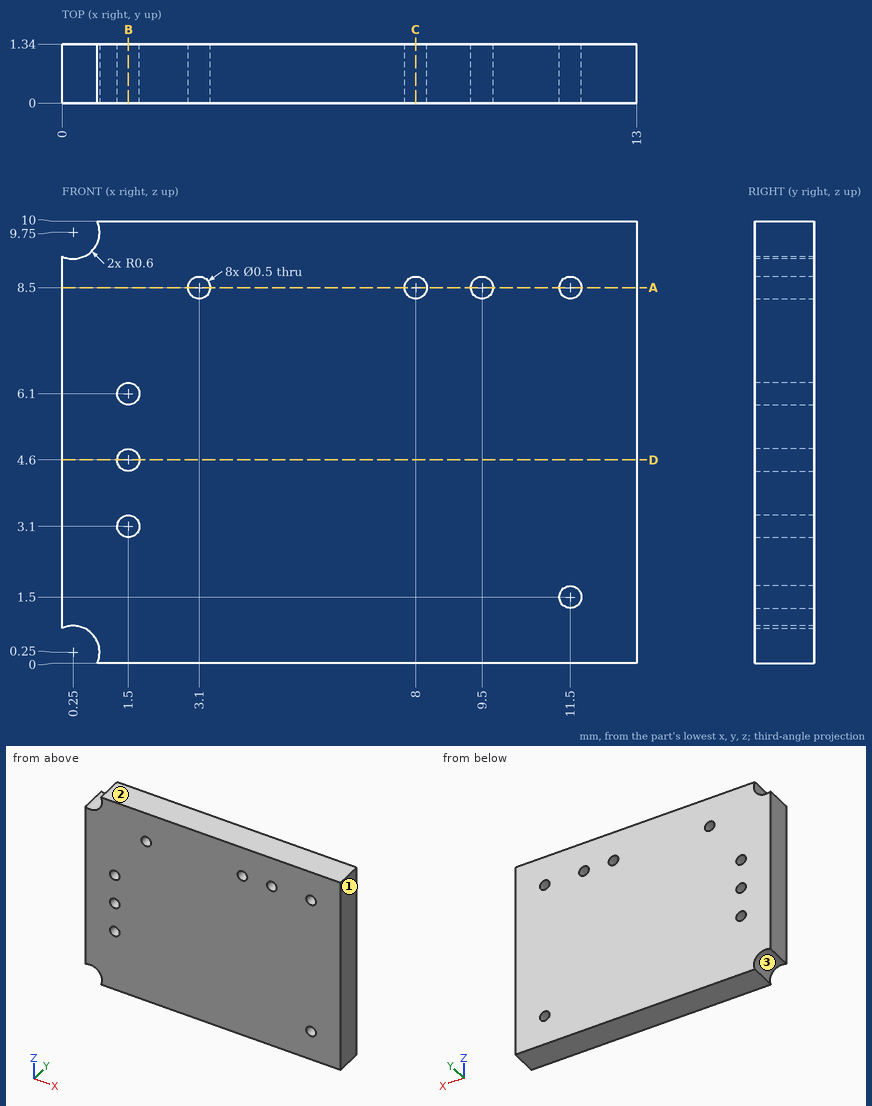
Answer from the drawing. Dimensions are ordinates in mm from the lowest x, y and z of the part. Round coordinates to 2 decimals unless told otherwise and drop trailing zeros. Write each loop counter-clockwise with the first axis right and the second up, starting at its lowest first coordinate (ties: lowest second). Pieces come first, ordered by that corner, then holes.
1. The part is cut by section D-D, the plane z = 4.6. Determine the outline of the cut face in (x, y), then the cut area to 4 significant figures.
2. The part is cut by section B-B, the plane x = 1.5. Determine the outline of the cut face in (y, z), then the cut area to 3 significant figures.
3. The part is cut by section A-A, the plane z = 8.5. Determine the outline of the cut face in (x, y).
4. The part is cut by section C-C, the plane x = 8. Determine the outline of the cut face in (y, z).
5. Straight lines are drawn through the part: L1, parallel to Z at x = 1.5, y = 0.5; L2, parallel to Z at x = 11.5, y = 0.8; L3, parallel to Z at x = 8, y = 0.95. For each, find the intervals that lie inside material, in ascending order.
6. Determine the mould class of the marked faces 1, 2 and 3 for opening direction Z: pulls with the +Z half, pulls with the -Z half, needs draft (parallel to the pull), parting line crosses it, or undercut.
Values:
1. outline: (0, 0) - (1.25, 0) - (1.25, 1.34) - (0, 1.34) - close; (1.75, 0) - (13, 0) - (13, 1.34) - (1.75, 1.34) - close
1. area: 16.75 mm2
2. outline: (0, 0) - (1.34, 0) - (1.34, 2.85) - (0, 2.85) - close; (0, 3.35) - (1.34, 3.35) - (1.34, 4.35) - (0, 4.35) - close; (0, 4.85) - (1.34, 4.85) - (1.34, 5.85) - (0, 5.85) - close; (0, 6.35) - (1.34, 6.35) - (1.34, 10) - (0, 10) - close
2. area: 11.4 mm2
3. outline: (0, 0) - (2.85, 0) - (2.85, 1.34) - (0, 1.34) - close; (3.35, 0) - (7.75, 0) - (7.75, 1.34) - (3.35, 1.34) - close; (8.25, 0) - (9.25, 0) - (9.25, 1.34) - (8.25, 1.34) - close; (9.75, 0) - (11.25, 0) - (11.25, 1.34) - (9.75, 1.34) - close; (11.75, 0) - (13, 0) - (13, 1.34) - (11.75, 1.34) - close
4. outline: (0, 0) - (1.34, 0) - (1.34, 8.25) - (0, 8.25) - close; (0, 8.75) - (1.34, 8.75) - (1.34, 10) - (0, 10) - close
5. L1: z = 0 to 2.85, 3.35 to 4.35, 4.85 to 5.85, 6.35 to 10
5. L2: z = 0 to 1.25, 1.75 to 8.25, 8.75 to 10
5. L3: z = 0 to 8.25, 8.75 to 10
6. face 1: needs draft
6. face 2: pulls with the +Z half
6. face 3: undercut
